from build123d import *
from build123d import SkipClean  # not in build123d's __all__

# Parameters (mm, degrees)
F1_DEPTH = 2.5
F2_W     = 3
F2_H     = 4.5
F3_DEPTH = 6.4
F4_R     = 1
F5_R     = 0.2


with BuildPart() as f1:
    # F0 (on Right) → F1 (new body)
    with BuildSketch(Plane.YZ):
        with BuildLine():
            ThreePointArc((-4.5, 4.5), (0, 0), (4.5, 4.5))
            Line((4.5, 4.5), (1.5, 4.5))
            ThreePointArc((1.5, 4.5), (0, 3), (-1.5, 4.5))
            Line((-1.5, 4.5), (-4.5, 4.5))
        make_face()
        with BuildLine():
            Line((1.5, 4.5), (4.5, 4.5))
            ThreePointArc((4.5, 4.5), (0, 9), (-4.5, 4.5))
            Line((-4.5, 4.5), (-1.5, 4.5))
            ThreePointArc((-1.5, 4.5), (0, 6), (1.5, 4.5))
        make_face()
        with BuildLine():
            Line((-4.5, -4.5), (4.5, -4.5))
            Line((4.5, -4.5), (4.5, 4.5))
            ThreePointArc((4.5, 4.5), (0, 0), (-4.5, 4.5))
            Line((-4.5, 4.5), (-4.5, -4.5))
        make_face()
    extrude(amount=F1_DEPTH)

    # F2 (on face) → F3 (join)
    with BuildSketch(Plane(origin=(0, 0, 0), x_dir=(0, -1, 0), z_dir=(-1, 0, 0))):
        with BuildLine():
            ThreePointArc((0.8237365529, 1.0983154039), (2.7507342597, 2.3358694512), (3.5, 4.5))
            ThreePointArc((3.5, 4.5), (-2.1641305488, 7.2507342597), (-0.8237365529, 1.0983154039))
            Line((-0.8237365529, 1.0983154039), (-1.5, 2))
            Line((-1.5, 2), (0, 2))
            Line((0, 2), (1.5, 2))
            Line((1.5, 2), (0.8237365529, 1.0983154039))
        make_face()
        with BuildLine():
            ThreePointArc((1.5, 4.5), (1.0606601718, 3.4393398282), (0, 3))
            ThreePointArc((0, 3), (-1.0606601718, 5.5606601718), (1.5, 4.5))
        make_face(mode=Mode.SUBTRACT)
        with BuildLine():
            Line((-1.5, 2), (-0.8237365529, 1.0983154039))
            ThreePointArc((-0.8237365529, 1.0983154039), (-0.4147914618, 1.0246657653), (0, 1))
            Line((0, 1), (0, 2))
            Line((0, 2), (-1.5, 2))
        make_face()
        with BuildLine():
            ThreePointArc((0, 1), (-0.4147914618, 1.0246657653), (-0.8237365529, 1.0983154039))
            Line((-0.8237365529, 1.0983154039), (0, 0))
            Line((0, 0), (0, 1))
        make_face()
        with BuildLine():
            Line((0, 0), (0.8237365529, 1.0983154039))
            ThreePointArc((0.8237365529, 1.0983154039), (0.4147914618, 1.0246657653), (0, 1))
            Line((0, 1), (0, 0))
        make_face()
        with BuildLine():
            ThreePointArc((0, 1), (0.4147914618, 1.0246657653), (0.8237365529, 1.0983154039))
            Line((0.8237365529, 1.0983154039), (1.5, 2))
            Line((1.5, 2), (0, 2))
            Line((0, 2), (0, 1))
        make_face()
        with Locations((-3, -2.25)):
            Rectangle(F2_W, F2_H)
        with Locations((3, -2.25)):
            Rectangle(F2_W, F2_H)
    with SkipClean():  # cleaning this boolean's faces spoils the solid; the shape is the same uncleaned
        extrude(amount=F3_DEPTH)

    # F4
    f4_edges = [f1.edges().sort_by_distance(p)[0] for p in [
        (-3.2, 1.5, 0),
        (-3.2, -1.5, 0),
        (-3.2, 0.823737, 1.098315),
        (-3.2, -0.823737, 1.098315),
    ]]
    fillet(f4_edges, radius=F4_R)

    # F5
    f5_edges = [f1.edges().sort_by_distance(p)[0] for p in [
        (-3.2, 0, 0),
    ]]
    fillet(f5_edges, radius=F5_R)


solid = f1.part
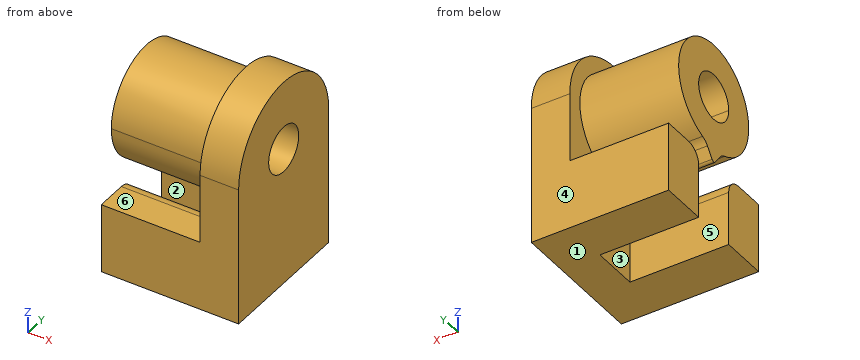
For this review, take the finished solid that the model builds, in its own axes (mm). Face numbers are marked on the shaded views. A direction names the side the tool comes from. Round coordinates to 2 decimals unless told otherwise and drop trailing zeros. Write each loop counter-clockwise with the first axis right and the second up, starting at its lowest first coordinate (ties: lowest second). Pieces come first, ordered by that corner, then holes. Notation, with made-up numbers: M 16.5,-37 L 67.5,-37 A21 ccw 67.5,-21 Z; hole C 71,86 d9. An arc over 180 degrees is marked long. Write item = value, one per line. Start each with the question number.
(1) The part is to be moulded in two halves that separate along Y. For the marked faces 4, 5 and 6, say which applies: +Y half, -Y half, draft (parallel to the pull), parting line (faces both ways), or undercut.
(2) We need section B-B (z = 4.75). Give the boundary of the cut face in (x, y), then the cut area to 3 significant figures.
(3) We need section D-D (y = 2.25). Give the boundary of the cut face in (x, z), then the cut area to 3 significant figures.
(4) Clearance check with flat-ended pins moving along their axes: pin 1 Ø3 at (x, y) = (-5, -1) entering from +Z; pin 2 Ø2 at (x, y) = (-1.5, -3.5) entering from +Z; pin 3 Ø1.6 at (x, y) = (-4, 3.5) entering from +Z. State where each tip first meets the part, or that it passes through.
(5) For the marked faces 1, 2 and 3, list the 3-axis set-ups (+Z, -Z, +X, -X, +Y, -Y) from which the entire face can be reached by the end or side of a thin tool; tool diameter is ignored.
(6) We need section C-C (x = 0.5). Give the boundary of the cut face in (y, z).
(7) We need section A-A (x = -0.5). Give the boundary of the cut face in (y, z).
(8) For line 1 along Y through (x, z) = (0.85, 4.5); line 2 along Z through (x, y) = (1.5, 0); line 3 along Z through (x, y) = (-3.75, 0), list the stretches that pass through material, from the lowest coordinate up.
Results found:
q1.face_4 = +Y half
q1.face_5 = undercut
q1.face_6 = draft
q2.outline = M -6.4,-3.49 L 0,-3.49 L 0,-4.49 L 2.5,-4.49 L 2.5,-1.48 L -6.4,-1.48 Z; M -6.4,1.48 L 2.5,1.48 L 2.5,4.49 L 0,4.49 L 0,3.49 L -6.4,3.49 Z
q2.area = 40.8 mm²
q3.outline = M -6.4,-4.5 L 2.5,-4.5 L 2.5,8.4 L 0,8.4 L 0,7.18 L -6.4,7.18 L -6.4,1.82 L 0,1.82 L 0,-0.03 L -6.4,-0.03 Z
q3.area = 95.2 mm²
q4.pin_1 = 8
q4.pin_2 = 6.95
q4.pin_3 = 6.73
q5.face_1 = -Z, +X, -X, +Y, -Y
q5.face_2 = -Z, -X
q5.face_3 = -X
q6.outline = M -4.5,-4.5 L 4.5,-4.5 L 4.5,4.5 A4.5 ccw -4.5,4.5 Z; hole C 0,4.5 d3
q7.outline = M -4.5,-4.5 L -1.5,-4.5 L -1.5,-1 A1 ccw -2.5,0 L -4.5,0 Z; M -1.11,1.18 A1 cw -0.62,0.83 L -0.16,0.21 A0.2 ccw 0.16,0.21 L 0.62,0.83 A1 cw 1.11,1.18 A3.5 ccw long Z; M 1.5,-4.5 L 4.5,-4.5 L 4.5,0 L 2.5,0 A1 ccw 1.5,-1 Z; hole C 0,4.5 d3
q8.line_1 = -4.5 to -1.5, 1.5 to 4.5
q8.line_2 = -4.5 to 3, 6 to 9
q8.line_3 = 0.13 to 3, 6 to 8
